Part model, mm, in its own coordinate system. Face numbers are marked on the shaded views. Give positions to 0.01 mm unless a question says otherwise; leave off trailing zeros. Write each loop counter-clockwise with the first axis right and the second up, starting at its lowest first coordinate (ties: lowest second). Pieces come first, ordered by that corner, then holes. Notation, with made-up numbers: M 65.5,57.25 L 75.5,57.25 A37 cw 75.5,96.25 Z; hole C -6.75,19 d8. An arc over 180 degrees is marked long. Use a Markdown table: item, result.
```python
from build123d import *

# Parameters (mm, degrees)
SKETCH1_R                        = 31.75
SKETCH1_R_2                      = 16.129
BOSS_EXTRUDE1_DEPTH              = 31.75
SKETCH2_W                        = 13.97
SKETCH2_H                        = 4.5
BOSS_EXTRUDE2_START              = -7.675
BOSS_EXTRUDE2_OUTLINE_R          = 31.75
BOSS_EXTRUDE2_OUTLINE_R_2        = 17.78
BOSS_EXTRUDE2_DEPTH              = 4.5
CUT_EXTRUDE2_REACH               = 56.993
CUT_EXTRUDE2_END_RADIUS          = 17.78
SKETCH8_R                        = 2
CUT_EXTRUDE3_REACH               = 56.993
CUT_EXTRUDE3_END_RADIUS          = 17.78
SKETCH9_R                        = 2
SKETCH10_R                       = 1
CUT_EXTRUDE4_DEPTH               = 10.141666667
TAP_DRILL_FOR_M5X0_8_TAP1_REACH  = 74.51
TAP_DRILL_FOR_M5X0_8_TAP1_BORE_R = 2.1


# Read off the part's stored shape, not the designer's step: Boss-Extrude2
with BuildPart() as part:
    # Sketch1 → Boss-Extrude1 (new body)
    with BuildSketch(Plane(origin=(0, 0, 0), x_dir=(1, 0, 0), z_dir=(0, 1, 0))):
        with Locations(Location((0, 0, 0), (0, 0, 270))):
            Circle(SKETCH1_R)
        with Locations(Location((0, 0, 0), (0, 0, 270))):
            Circle(SKETCH1_R_2, mode=Mode.SUBTRACT)
    extrude(amount=BOSS_EXTRUDE1_DEPTH)

    # Sketch2 → Cut-Revolve2 (revolve, cut)
    with BuildSketch(Plane.XY, mode=Mode.PRIVATE) as cut_revolve2_sk:
        with Locations((24.765, 26.325)):
            Rectangle(SKETCH2_W, SKETCH2_H)
        with Locations((24.765, 12.391666667)):
            Rectangle(SKETCH2_W, SKETCH2_H)
        with Locations((24.765, 5.425)):
            Rectangle(SKETCH2_W, SKETCH2_H)
        with Locations((24.765, 19.358333333)):
            Rectangle(SKETCH2_W, SKETCH2_H)
    revolve(cut_revolve2_sk.sketch.rotate(Axis((0, 0, 0), (0, 1, 0)), 90), axis=Axis((0, 0, 0), (0, 1, 0)), mode=Mode.SUBTRACT)

    # Boss-Extrude2 outline → Boss-Extrude2 (add)
    with BuildSketch(Plane(origin=(0, 31.75, 0), x_dir=(1, 0, 0), z_dir=(0, 1, 0)).offset(BOSS_EXTRUDE2_START)):
        Circle(BOSS_EXTRUDE2_OUTLINE_R)
        with BuildLine():
            ThreePointArc((18.265610967, -10.406997066), (18.915681572, -11.247857531), (19.33332562, -12.225206784))
            ThreePointArc((19.33332562, -12.225206784), (18.780593277, -11.327185978), (18.265610967, -10.406997066))
        make_face(mode=Mode.SUBTRACT)
        Circle(BOSS_EXTRUDE2_OUTLINE_R_2, mode=Mode.SUBTRACT)
    extrude(amount=BOSS_EXTRUDE2_DEPTH)

    # Cut-Extrude2: up to this cylinder (the profile starts inside it)
    cut_extrude2_end = Plane(origin=(0, 19.358333, 0), z_dir=(0, -1, 0)) * Cylinder(CUT_EXTRUDE2_END_RADIUS, 150.546, mode=Mode.PRIVATE)
    # Sketch8 → Cut-Extrude2 (cut, up to the surface)
    with BuildSketch(Plane.XY, mode=Mode.PRIVATE) as cut_extrude2_sk1:
        with Locations(Location((0, 19.358333333, 0), (0, 0, 180))):
            Circle(SKETCH8_R)
    cut_extrude2_tool1 = extrude(cut_extrude2_sk1.sketch, amount=CUT_EXTRUDE2_REACH, mode=Mode.PRIVATE) & cut_extrude2_end
    add(cut_extrude2_tool1.solids().sort_by_distance((0, 19.358333, 0))[0], mode=Mode.SUBTRACT)

    # Cut-Extrude3: up to this cylinder (the profile starts inside it)
    cut_extrude3_end = Plane(origin=(0, 19.358333, 0), z_dir=(0, -1, 0)) * Cylinder(CUT_EXTRUDE3_END_RADIUS, 150.546, mode=Mode.PRIVATE)
    # Sketch9 → Cut-Extrude3 (cut, up to the surface)
    with BuildSketch(Plane(origin=(0, 0, 0), x_dir=(0, 0, -1), z_dir=(1, 0, 0)), mode=Mode.PRIVATE) as cut_extrude3_sk1:
        with Locations((0, 19.358333333)):
            Circle(SKETCH9_R)
    cut_extrude3_tool1 = extrude(cut_extrude3_sk1.sketch, amount=-CUT_EXTRUDE3_REACH, mode=Mode.PRIVATE) & cut_extrude3_end
    add(cut_extrude3_tool1.solids().sort_by_distance((0, 19.358333, 0))[0], mode=Mode.SUBTRACT)

    # Sketch10 → Cut-Extrude4 (cut)
    with BuildSketch(Plane(origin=(0, 31.75, 0), x_dir=(1, 0, 0), z_dir=(0, 1, 0))):
        with Locations(Location((15.301734948, -13.370090036, 0), (0, 0, 270))):
            Circle(SKETCH10_R)
        with Locations(Location((13.370090036, 15.301734948, 0), (0, 0, 270))):
            Circle(SKETCH10_R)
        with Locations(Location((-15.301734948, 13.370090036, 0), (0, 0, 270))):
            Circle(SKETCH10_R)
        with Locations(Location((-13.370090036, -15.301734948, 0), (0, 0, 270))):
            Circle(SKETCH10_R)
    extrude(amount=-CUT_EXTRUDE4_DEPTH, mode=Mode.SUBTRACT)

    # Tap Drill for M5x0.8 Tap1 bore (on position points) → Tap Drill for M5x0.8 Tap1 (cut, up to next)
    with BuildSketch(Plane(origin=(15.301734948, 31.75, 13.370090036), x_dir=(0, 0, 1), z_dir=(0, 1, 0)), mode=Mode.PRIVATE) as tap_drill_for_m5x0_8_tap1_sk1:
        Circle(TAP_DRILL_FOR_M5X0_8_TAP1_BORE_R)
    tap_drill_for_m5x0_8_tap1_tool1 = extrude(tap_drill_for_m5x0_8_tap1_sk1.sketch, amount=-TAP_DRILL_FOR_M5X0_8_TAP1_REACH, mode=Mode.PRIVATE) & part.part
    # Tap Drill for M5x0.8 Tap1 bore (on position points) → Tap Drill for M5x0.8 Tap1 (cut, up to next)
    with BuildSketch(Plane(origin=(15.301734948, 31.75, 13.370090036), x_dir=(0, 0, 1), z_dir=(0, 1, 0)), mode=Mode.PRIVATE) as tap_drill_for_m5x0_8_tap1_sk2:
        with Locations((1.931644912, -28.671824984)):
            Circle(TAP_DRILL_FOR_M5X0_8_TAP1_BORE_R)
    tap_drill_for_m5x0_8_tap1_tool2 = extrude(tap_drill_for_m5x0_8_tap1_sk2.sketch, amount=-TAP_DRILL_FOR_M5X0_8_TAP1_REACH, mode=Mode.PRIVATE) & part.part
    # Tap Drill for M5x0.8 Tap1 bore (on position points) → Tap Drill for M5x0.8 Tap1 (cut, up to next)
    with BuildSketch(Plane(origin=(15.301734948, 31.75, 13.370090036), x_dir=(0, 0, 1), z_dir=(0, 1, 0)), mode=Mode.PRIVATE) as tap_drill_for_m5x0_8_tap1_sk3:
        with Locations((-26.740180072, -30.603469896)):
            Circle(TAP_DRILL_FOR_M5X0_8_TAP1_BORE_R)
    tap_drill_for_m5x0_8_tap1_tool3 = extrude(tap_drill_for_m5x0_8_tap1_sk3.sketch, amount=-TAP_DRILL_FOR_M5X0_8_TAP1_REACH, mode=Mode.PRIVATE) & part.part
    # Tap Drill for M5x0.8 Tap1 bore (on position points) → Tap Drill for M5x0.8 Tap1 (cut, up to next)
    with BuildSketch(Plane(origin=(15.301734948, 31.75, 13.370090036), x_dir=(0, 0, 1), z_dir=(0, 1, 0)), mode=Mode.PRIVATE) as tap_drill_for_m5x0_8_tap1_sk4:
        with Locations((-28.671824984, -1.931644912)):
            Circle(TAP_DRILL_FOR_M5X0_8_TAP1_BORE_R)
    tap_drill_for_m5x0_8_tap1_tool4 = extrude(tap_drill_for_m5x0_8_tap1_sk4.sketch, amount=-TAP_DRILL_FOR_M5X0_8_TAP1_REACH, mode=Mode.PRIVATE) & part.part
    add(tap_drill_for_m5x0_8_tap1_tool1.solids().sort_by_distance((15.301735, 31.75, 13.37009))[0], mode=Mode.SUBTRACT)
    add(tap_drill_for_m5x0_8_tap1_tool2.solids().sort_by_distance((-13.37009, 31.75, 15.301735))[0], mode=Mode.SUBTRACT)
    add(tap_drill_for_m5x0_8_tap1_tool3.solids().sort_by_distance((-15.301735, 31.75, -13.37009))[0], mode=Mode.SUBTRACT)
    add(tap_drill_for_m5x0_8_tap1_tool4.solids().sort_by_distance((13.37009, 31.75, -15.301735))[0], mode=Mode.SUBTRACT)


solid = part.part
```
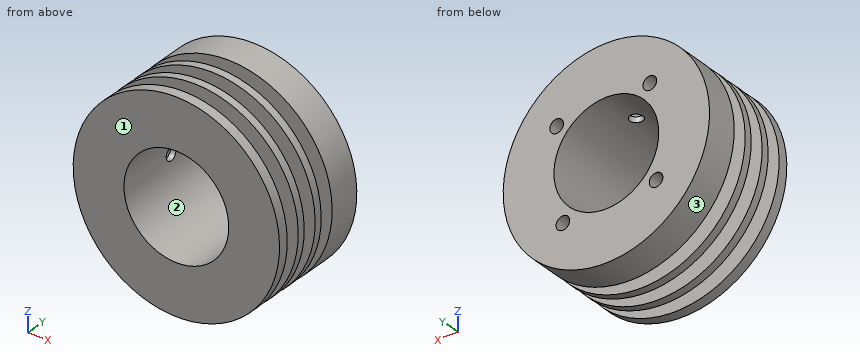
1. Drop flat-ended pins along their axis: P1, Ø10, axis at y = 22, z = -21.5, coming from the +X side; P2, Ø6, axis at y = 12.5, z = 20, coming from the -X side; P3, Ø12, axis at x = -25, y = 22.5, coming from the -Z side. Give the stop position or say it passes through.
Findings below:
| item | result |
|---|---|
| P1 | x = 27.13 |
| P2 | x = -26.22 |
| P3 | z = -25.44 |
2. Drill centre lines: L1, parallel to Y at x = 5.5, z = -23 (3 decimals); L2, parallel to Y at x = 0, z = 17.05; L3, parallel to X at y = 24, z = 12. Where is each one in solid material? Low to high.
Findings below:
| item | result |
|---|---|
| L1 | 0 to 3.175, 7.675 to 10.142, 14.642 to 17.108, 21.608 to 31.75 |
| L2 | 0 to 17.36, 21.36 to 31.75 |
| L3 | -29.39 to -10.78, 10.78 to 13.71, 16.89 to 29.39 |
3. Cut at C-C, the plane y = 16. Give the cut face in (x, z), then the cut area to 3 significant figures.
Findings below:
| item | result |
|---|---|
| outline | C 0,0 d63.5; hole C 0,0 d32.26 |
| area | 2,350 mm2 |
4. Cut at A-A, the plane x = -27. Give the cut face in (y, z) (3 decimals).
Findings below:
| item | result |
|---|---|
| outline | M 0,-16.705 L 3.175,-16.705 L 3.175,16.705 L 0,16.705 Z; M 7.675,-16.705 L 10.142,-16.705 L 10.142,16.705 L 7.675,16.705 Z; M 14.642,-16.705 L 17.108,-16.705 L 17.108,16.705 L 14.642,16.705 Z; M 21.608,-16.705 L 31.75,-16.705 L 31.75,16.705 L 21.608,16.705 Z |
5. Two-plate mould, pull along X, no slides. Class the marked faces 1, 2 and 3: released by +X, released by -X, zero draft, split by the parting line, or undercut.
Findings below:
| item | result |
|---|---|
| face 1 | zero draft |
| face 2 | undercut |
| face 3 | split by the parting line |
